from build123d import *

# Parameters (mm, degrees)
F1_DEPTH       = 2
F2_DEPTH       = 25
F3_R           = 2
F4_T1_DEPTH    = 4
F4_T3_DEPTH    = 4
F4_T5_DEPTH    = 4
F4_T7_DEPTH    = 17.2
F4_T9_DEPTH    = 17.2
F4_T11_DEPTH   = 4
F5_R           = 2
F6_SIZE        = 2
F8_D           = 3.3
F8_CSINK_D     = 6
F8_CSINK_ANGLE = 90


# Not quite as in the source:
# - a fillet or chamfer that OpenCascade refuses, or shapes differently, is made with other operations: its cross-section is extruded or revolved along the edge and cut away or added
# - a feature names something its author has since deleted; it is built from what else it names


with BuildPart() as f1:
    # F0 (on Top) → F1 (new body)
    with BuildSketch(Plane.XY):
        Polygon((28.2951036699, 0), (28.2951036699, 9.2), (4.9215265818, 9.2), (4.9215265818, 32.5735770881), (-4.2784734182, 32.5735770881), (-4.2784734182, 9.2), (-27.6520505063, 9.2), (-27.6520505063, 0), (-4.2784734182, 0), (-4.2784734182, -23.3735770881), (4.9215265818, -23.3735770881), (4.9215265818, 0), align=None)
        Polygon((4.9215265818, 9.2), (28.2951036699, 9.2), (28.2951036699, 13.2), (8.9215265818, 13.2), (8.9215265818, 32.5735770881), (4.9215265818, 32.5735770881), align=None)
        Polygon((28.2951036699, -4), (28.2951036699, 0), (4.9215265818, 0), (4.9215265818, -23.3735770881), (8.9215265818, -23.3735770881), (8.9215265818, -4), align=None)
        Polygon((-4.2784734182, 9.2), (-4.2784734182, 32.5735770881), (-8.2784734182, 32.5735770881), (-8.2784734182, 13.2), (-27.6520505063, 13.2), (-27.6520505063, 9.2), align=None)
        Polygon((-8.2784734182, -23.3735770881), (-4.2784734182, -23.3735770881), (-4.2784734182, 0), (-27.6520505063, 0), (-27.6520505063, -4), (-8.2784734182, -4), align=None)
    extrude(amount=F1_DEPTH)

    # F0 (on Top) → F2 (join)
    with BuildSketch(Plane.XY):
        Polygon((-4.2784734182, 9.2), (-4.2784734182, 32.5735770881), (-8.2784734182, 32.5735770881), (-8.2784734182, 13.2), (-27.6520505063, 13.2), (-27.6520505063, 9.2), align=None)
        Polygon((4.9215265818, 9.2), (28.2951036699, 9.2), (28.2951036699, 13.2), (8.9215265818, 13.2), (8.9215265818, 32.5735770881), (4.9215265818, 32.5735770881), align=None)
        Polygon((-8.2784734182, -23.3735770881), (-4.2784734182, -23.3735770881), (-4.2784734182, 0), (-27.6520505063, 0), (-27.6520505063, -4), (-8.2784734182, -4), align=None)
        Polygon((28.2951036699, -4), (28.2951036699, 0), (4.9215265818, 0), (4.9215265818, -23.3735770881), (8.9215265818, -23.3735770881), (8.9215265818, -4), align=None)
    extrude(amount=F2_DEPTH)

    # F3
    f3_edges = [f1.edges().sort_by_distance(p)[0] for p in [
        (8.921527, 13.2, 12.5),
        (8.921527, -4, 12.5),
    ]]
    fillet(f3_edges, radius=F3_R)

    # F4: fillet of radius 5 on 12 edges, made by hand

    # F4_s2 → F4_t1 (cut)
    with BuildSketch(Plane.XZ.offset(-13.2)):
        with BuildLine():
            ThreePointArc((23.2951036699, 25), (26.8306375758, 23.5355339059), (28.2951036699, 20))
            Line((28.2951036699, 20), (28.3951036699, 20))
            Line((28.3951036699, 20), (28.3951036699, 25.1))
            Line((28.3951036699, 25.1), (23.2951036699, 25.1))
            Line((23.2951036699, 25.1), (23.2951036699, 25))
        make_face()
        with BuildLine():
            ThreePointArc((-27.6520505063, 20), (-26.1875844123, 23.5355339059), (-22.6520505063, 25))
            Line((-22.6520505063, 25), (-22.6520505063, 25.1))
            Line((-22.6520505063, 25.1), (-27.7520505063, 25.1))
            Line((-27.7520505063, 25.1), (-27.7520505063, 20))
            Line((-27.7520505063, 20), (-27.6520505063, 20))
        make_face()
    extrude(amount=F4_T1_DEPTH, mode=Mode.SUBTRACT)

    # F4_s4 → F4_t3 (cut)
    with BuildSketch(Plane.YZ.offset(-8.2784734182)):
        with BuildLine():
            ThreePointArc((32.5735770881, 20), (31.1091109941, 23.5355339059), (27.5735770881, 25))
            Line((27.5735770881, 25), (27.5735770881, 25.1))
            Line((27.5735770881, 25.1), (32.6735770881, 25.1))
            Line((32.6735770881, 25.1), (32.6735770881, 20))
            Line((32.6735770881, 20), (32.5735770881, 20))
        make_face()
        with BuildLine():
            ThreePointArc((-23.3735770881, 20), (-21.9091109941, 23.5355339059), (-18.3735770881, 25))
            Line((-18.3735770881, 25), (-18.3735770881, 25.1))
            Line((-18.3735770881, 25.1), (-23.4735770881, 25.1))
            Line((-23.4735770881, 25.1), (-23.4735770881, 20))
            Line((-23.4735770881, 20), (-23.3735770881, 20))
        make_face()
    extrude(amount=F4_T3_DEPTH, mode=Mode.SUBTRACT)

    # F4_s6 → F4_t5 (cut)
    with BuildSketch(Plane.YZ.offset(4.9215265818)):
        with BuildLine():
            ThreePointArc((27.5735770881, 25), (31.1091109941, 23.5355339059), (32.5735770881, 20))
            Line((32.5735770881, 20), (32.6735770881, 20))
            Line((32.6735770881, 20), (32.6735770881, 25.1))
            Line((32.6735770881, 25.1), (27.5735770881, 25.1))
            Line((27.5735770881, 25.1), (27.5735770881, 25))
        make_face()
        with BuildLine():
            ThreePointArc((-18.3735770881, 25), (-21.9091109941, 23.5355339059), (-23.3735770881, 20))
            Line((-23.3735770881, 20), (-23.4735770881, 20))
            Line((-23.4735770881, 20), (-23.4735770881, 25.1))
            Line((-23.4735770881, 25.1), (-18.3735770881, 25.1))
            Line((-18.3735770881, 25.1), (-18.3735770881, 25))
        make_face()
    extrude(amount=F4_T5_DEPTH, mode=Mode.SUBTRACT)

    # F4_s8 → F4_t7 (cut)
    with BuildSketch(Plane.XZ.offset(-13.2)):
        with BuildLine():
            ThreePointArc((-22.6520505063, 0), (-26.1875844123, 1.4644660941), (-27.6520505063, 5))
            Line((-27.6520505063, 5), (-27.7520505063, 5))
            Line((-27.7520505063, 5), (-27.7520505063, -0.1))
            Line((-27.7520505063, -0.1), (-22.6520505063, -0.1))
            Line((-22.6520505063, -0.1), (-22.6520505063, 0))
        make_face()
        with BuildLine():
            ThreePointArc((28.2951036699, 5), (26.8306375758, 1.4644660941), (23.2951036699, 0))
            Line((23.2951036699, 0), (23.2951036699, -0.1))
            Line((23.2951036699, -0.1), (28.3951036699, -0.1))
            Line((28.3951036699, -0.1), (28.3951036699, 5))
            Line((28.3951036699, 5), (28.2951036699, 5))
        make_face()
    extrude(amount=F4_T7_DEPTH, mode=Mode.SUBTRACT)

    # F4_s10 → F4_t9 (cut)
    with BuildSketch(Plane.YZ.offset(-8.2784734182)):
        with BuildLine():
            ThreePointArc((27.5735770881, 0), (31.1091109941, 1.4644660941), (32.5735770881, 5))
            Line((32.5735770881, 5), (32.6735770881, 5))
            Line((32.6735770881, 5), (32.6735770881, -0.1))
            Line((32.6735770881, -0.1), (27.5735770881, -0.1))
            Line((27.5735770881, -0.1), (27.5735770881, 0))
        make_face()
        with BuildLine():
            ThreePointArc((-18.3735770881, 0), (-21.9091109941, 1.4644660941), (-23.3735770881, 5))
            Line((-23.3735770881, 5), (-23.4735770881, 5))
            Line((-23.4735770881, 5), (-23.4735770881, -0.1))
            Line((-23.4735770881, -0.1), (-18.3735770881, -0.1))
            Line((-18.3735770881, -0.1), (-18.3735770881, 0))
        make_face()
    extrude(amount=F4_T9_DEPTH, mode=Mode.SUBTRACT)

    # F4_s12 → F4_t11 (cut)
    with BuildSketch(Plane.XZ):
        with BuildLine():
            ThreePointArc((28.2951036699, 20), (26.8306375758, 23.5355339059), (23.2951036699, 25))
            Line((23.2951036699, 25), (23.2951036699, 25.1))
            Line((23.2951036699, 25.1), (28.3951036699, 25.1))
            Line((28.3951036699, 25.1), (28.3951036699, 20))
            Line((28.3951036699, 20), (28.2951036699, 20))
        make_face()
        with BuildLine():
            ThreePointArc((-27.6520505063, 20), (-26.1875844123, 23.5355339059), (-22.6520505063, 25))
            Line((-22.6520505063, 25), (-22.6520505063, 25.1))
            Line((-22.6520505063, 25.1), (-27.7520505063, 25.1))
            Line((-27.7520505063, 25.1), (-27.7520505063, 20))
            Line((-27.7520505063, 20), (-27.6520505063, 20))
        make_face()
    extrude(amount=F4_T11_DEPTH, mode=Mode.SUBTRACT)

    # F5
    f5_edges = [f1.edges().sort_by_distance(p)[0] for p in [
        (-8.278473, 13.2, 12.5),
        (-8.278473, -4, 12.5),
    ]]
    fillet(f5_edges, radius=F5_R)

    # F6
    f6_edges = [f1.edges().sort_by_distance(p)[0] for p in [
        (4.921527, 9.2, 13.5),
        (-4.278473, 9.2, 13.5),
        (4.921527, 0, 13.5),
        (-4.278473, 0, 13.5),
    ]]
    chamfer(f6_edges, length=F6_SIZE)

    # F8 (through all)
    with Locations(Plane(origin=(0, 0, 0), x_dir=(1, 0, 0), z_dir=(0, 0, -1))):
        with Locations((0, 10.087961331), (-15, -4.6), (15, -4.6), (0, -19.6)):
            CounterSinkHole(F8_D / 2, F8_CSINK_D / 2, counter_sink_angle=F8_CSINK_ANGLE)


solid = f1.part
Verification items for the finished model (mm, model axes). A direction names the side the tool comes from. Give positions to 0.01 mm unless a question says otherwise; leave off trailing zeros. Order: outer loops, then holes, each group sorted by start corner. A loop starts at its lowest first (then second) coordinate and runs counter-clockwise, first axis right, second up. Notation, with made-up numbers: M -16,6 L 36,6 A13 ccw 36,12 Z; hole C -23,49 d3. An arc over 180 degrees is marked long. Answer as a JSON object with one key per item and string values. Group by question number.
1) Cross-section at D-D (y = 23.5). Enter the section's corners in (x, z), then the cut area to 3 significant figures.
2) Cross-section at C-C (z = 13.5). Give the number of separate pieces and of enclosed holes in the cut face, then the cut area to 3 significant figures.
3) Depth check by flat-ended pin: pin 1 Ø8 at (y, z) = (23.5, 14) entering from -X; pin 2 Ø1.5 at (x, z) = (10.5, 11) entering from -Y; pin 3 Ø5.5 at (x, y) = (0, -10.09) entering from -Z. Enter the tip coordinate at first touch or a pass-through.
4) Access from +Z, -Z, +X, -X, +Y, -Y to the whole of each face (thin tool, end or side, straight path). Record for faces 1 (the face through (0, 7, 2)), 2 (the face through (-19, 13.2, 12)), 3 (the face through (8.922, 24, 12)).
5) Scan lines: line 1 along Y through (x, z) = (21, 13); line 2 along Y through (x, z) = (-15, 1.5); line 3 along X through (y, z) = (21.5, 9.5). Record each from-to range of solid material in increasing order. Write a range as [from, to].
6) Cross-section at B-B (x = 15). Enter the section's corners in (y, z).
7) Cross-section at A-A (x = 0). Enter the section's corners in (y, z).
8) Mould release check, pull along Y, two halves, no side actions. Record for faces 4 (the face through (9.492, 13.801, 12.325)), 5 (the face through (0.358, -8.477, 1.68)), 6 (the face through (4.922, 22, 13)): released by +Y, released by -Y, zero draft, split by the parting line, or undercut.
Result sheet:
{
 "1": {"outline": "M -8.28,0 L 8.92,0 L 8.92,25 L 4.92,25 L 4.92,2 L -4.28,2 L -4.28,25 L -8.28,25 Z", "area": "218 mm2"},
 "2": {"separate pieces": "4", "enclosed holes": "0", "area": "679 mm2"},
 "3": {"pin 1": "stops at x = -8.28", "pin 2": "stops at y = -4.38", "pin 3": "stops at z = 0.25"},
 "4": {"face 1": "+Z", "face 2": "+Z, -Z, -X, +Y", "face 3": "+Z, -Z, +X, +Y"},
 "5": {"line 1": "y = [-4, 0], [9.2, 13.2]", "line 2": "y = [-4, 2.95], [6.25, 13.2]", "line 3": "x = [-8.28, -4.28], [4.92, 8.92]"},
 "6": {"outline": "M -4,0 L 1.6,0 L 2.95,1.35 L 2.95,2 L 0,2 L 0,25 L -4,25 Z; M 6.25,1.35 L 7.6,0 L 13.2,0 L 13.2,25 L 9.2,25 L 9.2,2 L 6.25,2 Z"},
 "7": {"outline": "M -22.37,2 A5 ccw -18.37,0 L -13.09,0 L -11.74,1.35 L -11.74,2 Z; M -8.44,1.35 L -7.09,0 L 16.6,0 L 17.95,1.35 L 17.95,2 L -8.44,2 Z; M 21.25,1.35 L 22.6,0 L 27.57,0 A5 ccw 31.57,2 L 21.25,2 Z"},
 "8": {"face 4": "released by +Y", "face 5": "undercut", "face 6": "zero draft"}
}
